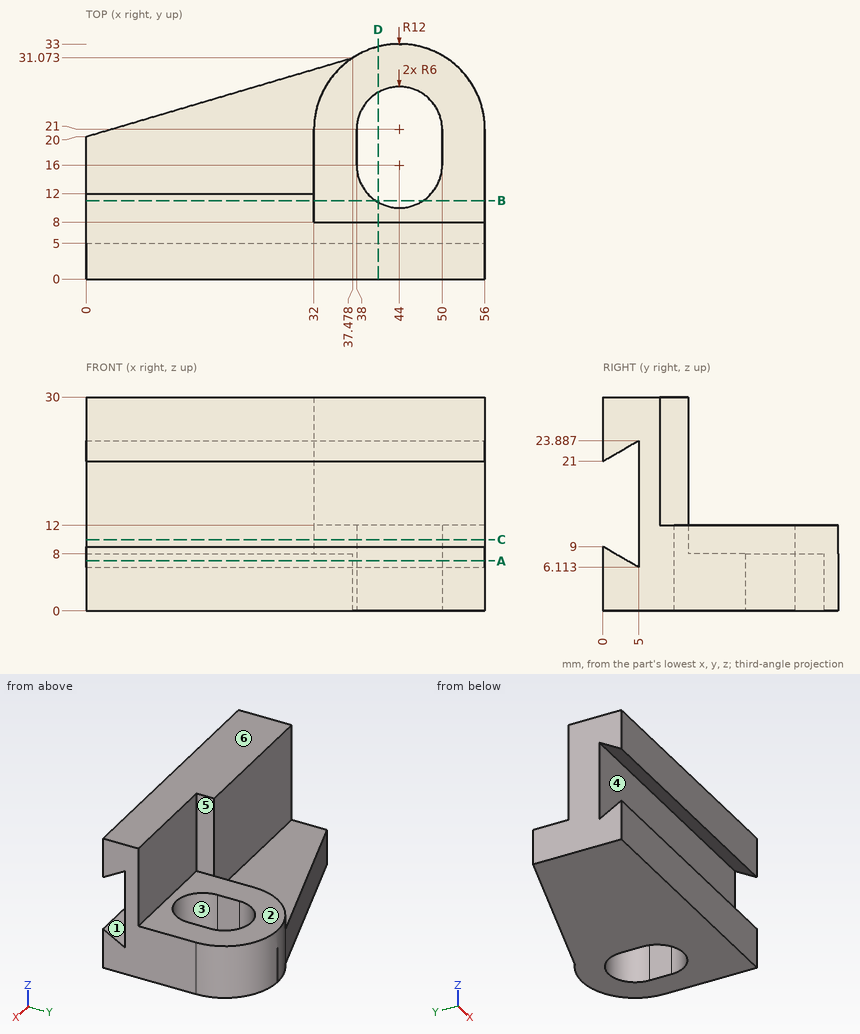
Print and shaded views of the part. All mm, measured from the part's lowest x, y and z. A direction names the side the tool comes from. Round coordinates to 2 decimals unless told otherwise and drop trailing zeros. Write each loop counter-clockwise with the first axis right and the second up, starting at its lowest first coordinate (ties: lowest second). Pieces come first, ordered by that corner, then holes.
(1) Slice it at C-C, the plane z = 10. Write the cut outline in (x, y), and give its area (3 significant figures).
(2) Slice it at D-D, the plane x = 41. Write the cut outline in (y, z).
(3) Mould opens along Z. For the marked faces 4, 5 and 6 say: pulls with the +Z half, pulls with the -Z half, needs draft (parallel to the pull), parting line crosses it, or undercut.
(4) Drop flat-ended pins along their axis: P1, Ø3, axis at y = 10.5, z = 19.5, coming from the +X side; P2, Ø1, axis at x = 44, z = 24, coming from the +Y side; P3, Ø2, axis at y = 16, z = 9.5, coming from the -X side; P4, Ø7, axis at x = 43.5, y = 20.5, coming from the +Z side. Give the stop position or say it passes through.
(5) Slice it at A-A, the plane z = 7. Count the separate pieces of the cut face and the enclosed holes in it, and give its area (3 significant figures).
(6) 3-axis set-ups, long thin cutter, end or side, ignore diameter. For the marked faces 1, 2 and 3: which of +Z, -Z, +X, -X, +Y, -Y reach the whole face in a straight line?
(7) Slice it at B-B, the plane y = 11. Write the cut outline in (x, z), and give its area (3 significant figures).
(8) Probe line 1 along X through (y, z) = (10, 25.5); line 2 along Y through (x, z) = (4, 24.75); line 3 along Y through (x, z) = (24, 7.75) (1 decimal). List the from-to ranges inside material, lowest first.
From the geometry:
1. outline: (0, 5) - (56, 5) - (56, 21) arc R12 ccw to (32, 21) - (32, 12) - (0, 12) - close; hole (38, 16) arc R6 ccw to (50, 16) - (50, 21) arc R6 ccw to (38, 21) - close
1. area: 661 mm2
2. outline: (0, 0) - (10.8, 0) - (10.8, 12) - (8, 12) - (8, 30) - (0, 30) - (0, 21) - (5, 23.89) - (5, 6.11) - (0, 9) - close; (26.2, 0) - (32.62, 0) - (32.62, 12) - (26.2, 12) - close
3. face 4: undercut
3. face 5: needs draft
3. face 6: pulls with the +Z half
4. P1: stops at x = 32
4. P2: stops at y = 8
4. P3: stops at x = 32
4. P4: passes through
5. separate pieces: 2
5. enclosed holes: 1
5. area: 1,270 mm2
6. face 1: +X, -X
6. face 2: +Z, +X, +Y
6. face 3: +Z, -Z
7. outline: (0, 0) - (40.68, 0) - (40.68, 12) - (32, 12) - (32, 30) - (0, 30) - close; (47.32, 0) - (56, 0) - (56, 12) - (47.32, 12) - close
7. area: 1,170 mm2
8. line 1: x = 0 to 32
8. line 2: y = 0 to 12
8. line 3: y = 0 to 2.2, 5 to 27.1
